Geometry check sheet. Reference: the model listing, model coordinates, mm. A direction names the side the tool comes from. Coordinates: 2 decimals unless noted, no trailing zeros. Order: outer loops, then holes, each group sorted by start corner. A loop starts at its lowest first (then second) coordinate and runs counter-clockwise, first axis right, second up.
```python
from build123d import *

# Parameters (mm, degrees)
F1_DEPTH = 12.7


with BuildPart() as f1:
    # F0 (on Top) → F1 (new body)
    with BuildSketch(Plane.XY):
        with BuildLine():
            Line((3.302, 0), (-3.302, 0))
            ThreePointArc((-3.302, 0), (-3.851926, 0.3175), (-3.851926, 0.9525))
            Line((-3.851926, 0.9525), (-3.175, 2.12497))
            Line((-3.175, 2.12497), (-3.175, 4.445))
            ThreePointArc((-3.175, 4.445), (-3.360987, 4.894013), (-3.81, 5.08))
            Line((-3.81, 5.08), (-4.910715, 5.08))
            ThreePointArc((-4.910715, 5.08), (-5.297279, 4.948779), (-5.524078, 4.60935))
            Line((-5.524078, 4.60935), (-6.368814, 1.45675))
            ThreePointArc((-6.368814, 1.45675), (-5.820897, -1.297818), (-3.302, -2.54))
            Line((-3.302, -2.54), (15.24, -2.54))
            ThreePointArc((15.24, -2.54), (16.51, -1.27), (15.24, 0))
            Line((15.24, 0), (9.005439, 0))
            ThreePointArc((9.005439, 0), (8.243439, 0.204177), (7.685616, 0.762))
            Line((7.685616, 0.762), (5.375926, 4.7625))
            ThreePointArc((5.375926, 4.7625), (5.1435, 4.994926), (4.826, 5.08))
            Line((4.826, 5.08), (3.81, 5.08))
            ThreePointArc((3.81, 5.08), (3.360987, 4.894013), (3.175, 4.445))
            Line((3.175, 4.445), (3.175, 2.12497))
            Line((3.175, 2.12497), (3.851926, 0.9525))
            ThreePointArc((3.851926, 0.9525), (3.851926, 0.3175), (3.302, 0))
        make_face()
    extrude(amount=F1_DEPTH)


solid = f1.part
```
Item 1: Release check for a two-part mould opening along X. For faces 1 (the face through (8.25, 0.2, 6.26)), 2 (the face through (3.509, 1.547, 6.261)), 3 (the face through (5, 0, 12.7)) record: pulls with the +X half, pulls with the -X half, needs draft (parallel to the pull), parting line crosses it, or undercut.
Item 2: Depth check by flat-ended pin: P1, Ø1, axis at y = 4, z = 2.5, coming from the -X side; P2, Ø3, axis at y = 2, z = 4.5, coming from the +X side; P3, Ø3, axis at x = 11, z = 8.5, coming from the +Y side; P4, Ø2, axis at x = 0, y = 1.5, coming from the -Z side. Enter the tip coordinate at first touch or a pass-through.
Item 3: Tool access check on faces 4 (the face through (3.86, 0.33, 6.26)), 5 (the face through (12, 0, 6)), 6 (the face through (3.175, 3, 6)), 7 (the face through (6, -2.54, 6)), 8 (the face through (16.51, -1.3, 6.26)). Record the directions out of +Z, -Z, +X, -X, +Y, -Y that give a thin tool (end or side, any length) a straight path to the whole face; none if there is none.
Item 4: Sectioned sample at D-D (y = -1.27). Record the cut outline in (x, z).
Item 5: Sectioned sample at C-C (x = 1.25). Record the cut outline in (y, z), and give its area (3 significant figures).
Item 6: Sectioned sample at B-B (y = 3). Record the cut outline in (x, z) (1 decimal).
Item 7: Thickness scan on line 1 along Y through (x, z) = (2, 4.25); line 2 along X through (y, z) = (3.25, 10.75) (3 decimals); line 3 along X through (y, z) = (4, 10.25) (3 decimals). Record the ranges inside material, lowest first.
Geometry check:
1. face 1: pulls with the +X half
1. face 2: undercut
1. face 3: needs draft
2. P1: stops at x = -5.82
2. P2: stops at x = 7.88
2. P3: stops at y = 0
2. P4: passes through
3. face 4: +Z, -Z
3. face 5: +Z, -Z, +X, +Y
3. face 6: +Z, -Z, +Y
3. face 7: +Z, -Z, +X, -X, -Y
3. face 8: +Z, -Z, +X
4. outline: (-5.84, 0) - (16.51, 0) - (16.51, 12.7) - (-5.84, 12.7) - close
5. outline: (-2.54, 0) - (0, 0) - (0, 12.7) - (-2.54, 12.7) - close
5. area: 32.3 mm2
6. outline: (-6, 0) - (-3.2, 0) - (-3.2, 12.7) - (-6, 12.7) - close; (3.2, 0) - (6.4, 0) - (6.4, 12.7) - (3.2, 12.7) - close
7. line 1: y = -2.54 to 0
7. line 2: x = -5.888 to -3.175, 3.175 to 6.249
7. line 3: x = -5.687 to -3.175, 3.175 to 5.816
